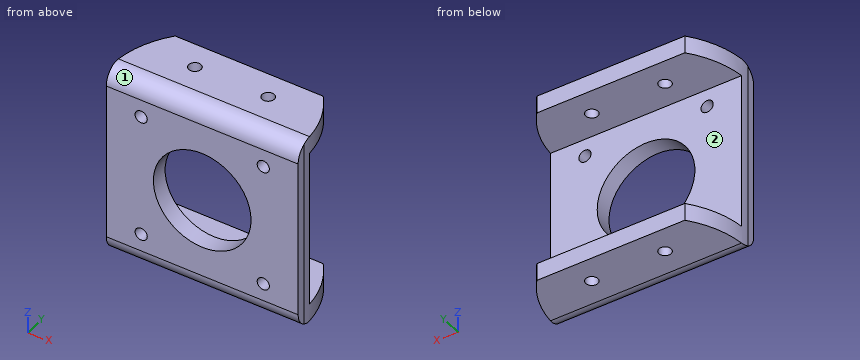
```python
from build123d import *

# Parameters (mm, degrees)
SKETCH1_W           = 55
SKETCH1_H           = 55
BOSS_EXTRUDE1_DEPTH = 5
CUT_EXTRUDE2_REACH  = 7
SKETCH10_R          = 14
SKETCH10_R_2        = 1.75
SKETCH11_W          = 55
SKETCH11_H          = 5
BOSS_EXTRUDE2_DEPTH = 15
FILLET1_R           = 5
SKETCH12_R          = 1.75
CUT_EXTRUDE3_DEPTH  = 56
CUT_EXTRUDE4_DEPTH  = 56


with BuildPart() as part:
    # Sketch1 → Boss-Extrude1 (new body)
    with BuildSketch(Plane(origin=(0, 0, 0), x_dir=(1, 0, 0), z_dir=(0, 1, 0))):
        Rectangle(SKETCH1_W, SKETCH1_H)
    extrude(amount=BOSS_EXTRUDE1_DEPTH)

    # Sketch10 → Cut-Extrude2 (cut, up to next)
    with BuildSketch(Plane(origin=(0, 5, 0), x_dir=(1, 0, 0), z_dir=(0, 1, 0)), mode=Mode.PRIVATE) as cut_extrude2_sk1:
        Circle(SKETCH10_R)
    cut_extrude2_tool1 = extrude(cut_extrude2_sk1.sketch, amount=-CUT_EXTRUDE2_REACH, mode=Mode.PRIVATE) & part.part
    add(cut_extrude2_tool1.solids().sort_by_distance((0, 5, 0))[0], mode=Mode.SUBTRACT)
    # Sketch10 → Cut-Extrude2 (cut, up to next)
    with BuildSketch(Plane(origin=(0, 5, 0), x_dir=(1, 0, 0), z_dir=(0, 1, 0)), mode=Mode.PRIVATE) as cut_extrude2_sk2:
        with Locations((-17.5, 17.5)):
            Circle(SKETCH10_R_2)
    cut_extrude2_tool2 = extrude(cut_extrude2_sk2.sketch, amount=-CUT_EXTRUDE2_REACH, mode=Mode.PRIVATE) & part.part
    add(cut_extrude2_tool2.solids().sort_by_distance((-17.5, 5, -17.5))[0], mode=Mode.SUBTRACT)
    # Sketch10 → Cut-Extrude2 (cut, up to next)
    with BuildSketch(Plane(origin=(0, 5, 0), x_dir=(1, 0, 0), z_dir=(0, 1, 0)), mode=Mode.PRIVATE) as cut_extrude2_sk3:
        with Locations((17.5, 17.5)):
            Circle(SKETCH10_R_2)
    cut_extrude2_tool3 = extrude(cut_extrude2_sk3.sketch, amount=-CUT_EXTRUDE2_REACH, mode=Mode.PRIVATE) & part.part
    add(cut_extrude2_tool3.solids().sort_by_distance((17.5, 5, -17.5))[0], mode=Mode.SUBTRACT)
    # Sketch10 → Cut-Extrude2 (cut, up to next)
    with BuildSketch(Plane(origin=(0, 5, 0), x_dir=(1, 0, 0), z_dir=(0, 1, 0)), mode=Mode.PRIVATE) as cut_extrude2_sk4:
        with Locations((17.5, -17.5)):
            Circle(SKETCH10_R_2)
    cut_extrude2_tool4 = extrude(cut_extrude2_sk4.sketch, amount=-CUT_EXTRUDE2_REACH, mode=Mode.PRIVATE) & part.part
    add(cut_extrude2_tool4.solids().sort_by_distance((17.5, 5, 17.5))[0], mode=Mode.SUBTRACT)
    # Sketch10 → Cut-Extrude2 (cut, up to next)
    with BuildSketch(Plane(origin=(0, 5, 0), x_dir=(1, 0, 0), z_dir=(0, 1, 0)), mode=Mode.PRIVATE) as cut_extrude2_sk5:
        with Locations((-17.5, -17.5)):
            Circle(SKETCH10_R_2)
    cut_extrude2_tool5 = extrude(cut_extrude2_sk5.sketch, amount=-CUT_EXTRUDE2_REACH, mode=Mode.PRIVATE) & part.part
    add(cut_extrude2_tool5.solids().sort_by_distance((-17.5, 5, 17.5))[0], mode=Mode.SUBTRACT)

    # Sketch11 → Boss-Extrude2 (add)
    with BuildSketch(Plane(origin=(0, 5, 0), x_dir=(1, 0, 0), z_dir=(0, 1, 0))):
        with Locations((0, 25)):
            Rectangle(SKETCH11_W, SKETCH11_H)
        with Locations((0, -25)):
            Rectangle(SKETCH11_W, SKETCH11_H)
    extrude(amount=BOSS_EXTRUDE2_DEPTH)

    # Fillet1
    fillet1_edges = [part.edges().sort_by_distance(p)[0] for p in [
        (0, 0, 27.5),
        (0, 0, -27.5),
    ]]
    fillet(fillet1_edges, radius=FILLET1_R)

    # Sketch12 → Cut-Extrude3 (cut, through all)
    with BuildSketch(Plane(origin=(0, 0, -27.5), x_dir=(-1, 0, 0), z_dir=(0, 0, -1))):
        with Locations((-10.5, 12.5)):
            Circle(SKETCH12_R)
        with Locations((10.5, 12.5)):
            Circle(SKETCH12_R)
    extrude(amount=-CUT_EXTRUDE3_DEPTH, mode=Mode.SUBTRACT)

    # Sketch13 → Cut-Extrude4 (cut, through all)
    with BuildSketch(Plane.XY.offset(27.5)):
        with BuildLine():
            Line((-27.5, 2.5), (-27.5, 20))
            Line((-27.5, 20), (-21.213203436, 20))
            ThreePointArc((-21.213203436, 20), (-25.880621075, 11.797497123), (-27.5, 2.5))
        make_face()
        with BuildLine():
            Line((21.213203436, 20), (27.5, 20))
            Line((27.5, 20), (27.5, 2.5))
            ThreePointArc((27.5, 2.5), (25.880621075, 11.797497123), (21.213203436, 20))
        make_face()
    extrude(amount=-CUT_EXTRUDE4_DEPTH, mode=Mode.SUBTRACT)


solid = part.part
```
The listing builds one solid part. Answer for the finished solid, in the listing's coordinates (mm). Face numbers are marked on the shaded views. A direction names the side the tool comes from. Give positions to 0.01 mm unless a question says otherwise; leave off trailing zeros. Order: outer loops, then holes, each group sorted by start corner. A loop starts at its lowest first (then second) coordinate and runs counter-clockwise, first axis right, second up.
1) Find section B-B on z = -17.5. Write down the section's boundary in (x, y).
Reported:
outline: (-27.5, 0) - (-19.25, 0) - (-19.25, 5) - (-27.39, 5) arc R27.5 ccw to (-27.5, 2.5) - close; (-15.75, 0) - (15.75, 0) - (15.75, 5) - (-15.75, 5) - close; (19.25, 0) - (27.5, 0) - (27.5, 2.5) arc R27.5 ccw to (27.39, 5) - (19.25, 5) - close
2) Given P1, Ø3, axis at x = 17.5, z = -17.5, coming from the -Y side (1 decimal); P2, Ø5, axis at y = 5.5, z = -15.5, coming from the -X side; P3, Ø2, axis at y = 4.5, z = -7.5, coming from the +X side; P4, Ø4, axis at x = 17.5, z = 17.5, coming from the +Y side, each flat-ended and moving along its own axis, determine where each tip first touches the part or whether it passes through.
Reported:
P1: passes through
P2: stops at x = -27.5
P3: stops at x = 27.48
P4: stops at y = 5
3) Find section A-A on x = 0. Write down the section's boundary in (y, z), then the cut area to 3 significant figures.
Reported:
outline: (0, -22.5) arc R5 ccw to (5, -27.5) - (20, -27.5) - (20, -22.5) - (5, -22.5) - (5, -14) - (0, -14) - close; (0, 14) - (5, 14) - (5, 22.5) - (20, 22.5) - (20, 27.5) - (5, 27.5) arc R5 ccw to (0, 22.5) - close
area: 274 mm2
4) For the marked faces 1 and 2, determine the directions among +Z, -Z, +X, -X, +Y, -Y from which every point of the face is accessible in a straight line to the end or side of a thin tool.
Reported:
face 1: +Z, +X, -X, -Y
face 2: +X, -X, +Y
5) Find section D-D on x = 17.5. Write down the section's boundary in (y, z).
Reported:
outline: (0, -22.5) arc R5 ccw to (5, -27.5) - (20, -27.5) - (20, -22.5) - (5, -22.5) - (5, -19.25) - (0, -19.25) - close; (0, -15.75) - (5, -15.75) - (5, 15.75) - (0, 15.75) - close; (0, 19.25) - (5, 19.25) - (5, 22.5) - (20, 22.5) - (20, 27.5) - (5, 27.5) arc R5 ccw to (0, 22.5) - close
6) Find section C-C on y = 7.25. Write down the section's boundary in (x, z), then the cut area to 3 significant figures.
Reported:
outline: (-27.09, -27.5) - (27.09, -27.5) - (27.09, -22.5) - (-27.09, -22.5) - close; (-27.09, 22.5) - (27.09, 22.5) - (27.09, 27.5) - (-27.09, 27.5) - close
area: 542 mm2
7) Consider line 1 along X through (y, z) = (1.1, -17.5); line 2 along Z through (x, y) = (11, 10); line 3 along X through (y, z) = (13.5, 23.5). Determine where each line is inside the solid, lowest interval first.
Reported:
line 1: x = -27.5 to -19.25, -15.75 to 15.75, 19.25 to 27.5
line 2: z = -27.5 to -22.5, 22.5 to 27.5
line 3: x = -25.2 to -11.94, -9.06 to 9.06, 11.94 to 25.2
